from build123d import *

# Parameters (mm, degrees)
EXTRUDE_1_DEPTH     = 17
SKETCH_2_R          = 8.75
EXTRUDE_2_DEPTH     = 3
SKETCH_3_R          = 10
EXTRUDE_3_DEPTH     = 12.5
CHAMFER_1_SIZE      = 1.5
SKETCH_6_R          = 7
CUT_EXTRUDE_1_DEPTH = 37.958912269
CHAMFER_2_SIZE      = 0.5
SKETCH_7_R          = 9.5
CUT_EXTRUDE_2_DEPTH = 13


with BuildPart() as part:
    # 草图1 → 凸台-拉伸1 (new body)
    with BuildSketch(Plane(origin=(0, 0, 0), x_dir=(1, 0, 0), z_dir=(0, 1, 0))):
        Polygon((6.553289027, 11.549360859), (-6.725395388, 11.449995205), (-13.278684415, -0.099365654), (-6.553289027, -11.549360859), (6.725395388, -11.449995205), (13.278684415, 0.099365654), align=None)
    extrude(amount=EXTRUDE_1_DEPTH)

    # 草图2 → 凸台-拉伸2 (add)
    with BuildSketch(Plane(origin=(0, 17, 0), x_dir=(1, 0, 0), z_dir=(0, 1, 0))):
        with Locations(Location((0, 0, 0), (0, 0, 270))):
            Circle(SKETCH_2_R)
    extrude(amount=EXTRUDE_2_DEPTH)

    # 草图3 → 凸台-拉伸3 (add)
    with BuildSketch(Plane(origin=(0, 20, 0), x_dir=(1, 0, 0), z_dir=(0, 1, 0))):
        with Locations(Location((0, 0, 0), (0, 0, 270))):
            Circle(SKETCH_3_R)
    extrude(amount=EXTRUDE_3_DEPTH)

    # 倒角1
    chamfer_1_edges = [part.edges().sort_by_distance(p)[0] for p in [
        (0, 32.5, -10),
    ]]
    chamfer(chamfer_1_edges, length=CHAMFER_1_SIZE)

    # 草图5 → 切除-旋转3 (revolve, cut)
    with BuildSketch(Plane(origin=(0, 0, 0), x_dir=(0.49350563267132574, 0, -0.8697426001534446), z_dir=(0.8697426001534445, 0, 0.4935056326713257)), mode=Mode.PRIVATE) as cut_revolve_3_sk:
        Polygon((13.279056191, 1), (11.279056191, 0), (13.279056191, 0), align=None)
    revolve(cut_revolve_3_sk.sketch.rotate(Axis((0, -1000, 0), (0, 1, 0)), 180.000000003), axis=Axis((0, -1000, 0), (0, 1, 0)), mode=Mode.SUBTRACT)

    # 草图6 → 切除-拉伸1 (cut, through all)
    with BuildSketch(Plane(origin=(0, 32.5, 0), x_dir=(1, 0, 0), z_dir=(0, 1, 0))):
        with Locations(Location((0, 0, 0), (0, 0, 270))):
            Circle(SKETCH_6_R)
    extrude(amount=-CUT_EXTRUDE_1_DEPTH, mode=Mode.SUBTRACT)

    # 倒角2
    chamfer_2_edges = [part.edges().sort_by_distance(p)[0] for p in [
        (0, 0, -7),
        (0, 32.5, -7),
    ]]
    chamfer(chamfer_2_edges, length=CHAMFER_2_SIZE)

    # 草图7 → 切除-拉伸2 (cut)
    with BuildSketch(Plane.XZ):
        with Locations(Location((0, 0, 0), (0, 0, 270))):
            Circle(SKETCH_7_R)
    extrude(amount=-CUT_EXTRUDE_2_DEPTH, mode=Mode.SUBTRACT)


solid = part.part
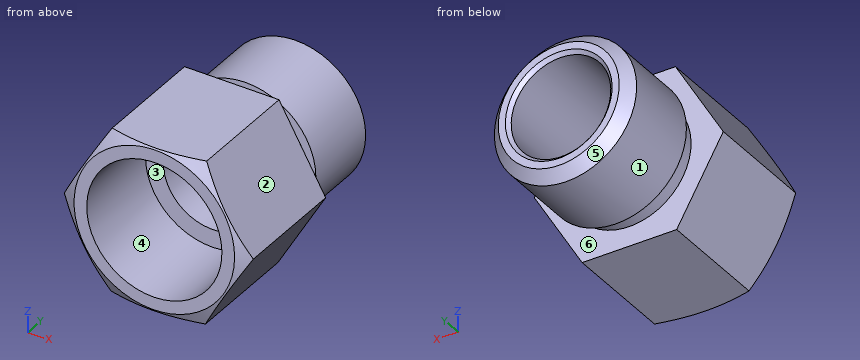
Here's how the part is built. I have some questions about the finished solid (model axes, mm). Face numbers are marked on the shaded views. A direction names the side the tool comes from. Give positions to 0.01 mm unless a question says otherwise; leave off trailing zeros. Loops run counter-clockwise (first coordinate to the right, second up) from the corner with the lowest first, then second, coordinate; pieces in that order, holes last. Notation, with made-up numbers: (59, 86) -> (117, 86) arc R22 ccw to (117, 98) -> close; hole circle Ø11 at (84.5, 40.5). An arc over 180 degrees is marked (long way). Answer as a JSON object with one key per item and string values. Group by question number.
Item 1: On a 3-axis mill with a long thin cutter (end or side, diameter ignored), from which of +Z, -Z, +X, -X, +Y, -Y can I reach the whole of each face in a straight line? I mean the marked faces 1, 2 and 3. Say none if no direction works.
Item 2: Imagine slicing it at B-B on x = 0. Write out the boundary of the cut face in (y, z), then the cut area to 3 significant figures.
Item 3: Thinking about a two-plate mould opening in Z: for the marked faces 4, 5 and 6, which applies, pulls with the +Z half, pulls with the -Z half, needs draft (parallel to the pull), parting line crosses it, or undercut?
Item 4: Will these pins go through, and if not, where does the flat tip stop? pin 1 (2 mm diameter, centred on y = 6, z = 2.5, fed in from -X); pin 2 (1 mm diameter, centred on y = 21.5, z = -1, fed in from -X); pin 3 (1 mm diameter, centred on x = -10.5, z = 8.5, fed in from +Y); pin 4 (1.5 mm diameter, centred on y = 4, z = 4.5, fed in from -X).
Item 5: Imagine slicing it at C-C on y = 26. Write out the boundary of the cut face in (x, z), then the cut area to 3 significant figures.
Item 6: I need wall thicknesses on L1, parallel to X at y = 20.25, z = 0; L2, parallel to Z at x = 3.5, y = 3; L3, parallel to Z at x = -7.25, y = 7. Which ranges of each line are inside material? Lowest first, please.
Item 7: Imagine slicing it at A-A on y = 2.5. Write out the boundary of the cut face in (x, z).
Answer list:
{
 "1": {"face 1": "+Y", "face 2": "+Z, +X, +Y, -Y", "face 3": "-Y"},
 "2": {"outline": "(0, -11.28) -> (0.11, -11.5) -> (17, -11.5) -> (17, -8.75) -> (20, -8.75) -> (20, -10) -> (31, -10) -> (32.5, -8.5) -> (32.5, -7.5) -> (32, -7) -> (13, -7) -> (13, -9.5) -> (0, -9.5) -> close; (0, 9.5) -> (13, 9.5) -> (13, 7) -> (32, 7) -> (32.5, 7.5) -> (32.5, 8.5) -> (31, 10) -> (20, 10) -> (20, 8.75) -> (17, 8.75) -> (17, 11.5) -> (0.11, 11.5) -> (0, 11.28) -> close", "area": "171 mm2"},
 "3": {"face 4": "undercut", "face 5": "parting line crosses it", "face 6": "needs draft"},
 "4": {"pin 1": "stops at x = -12.46", "pin 2": "stops at x = -9.99", "pin 3": "passes through", "pin 4": "stops at x = -11.13"},
 "5": {"outline": "circle Ø20 at (0, 0); hole circle Ø14 at (0, 0)", "area": "160 mm2"},
 "6": {"L1": "x = -10 to -7, 7 to 10", "L2": "z = -11.53 to -8.83, 8.83 to 11.47", "L3": "z = -10.53 to -6.14, 6.14 to 10.36"},
 "7": {"outline": "(-13.28, 0.1) -> (-6.73, -11.45) -> (6.55, -11.55) -> (13.28, -0.1) -> (6.73, 11.45) -> (-6.55, 11.55) -> close; hole circle Ø19 at (0, 0)"}
}
